Part model, mm, in its own coordinate system. A direction names the side the tool comes from. Give positions to 0.01 mm unless a question says otherwise; leave off trailing zeros. Write each loop counter-clockwise with the first axis right and the second up, starting at its lowest first coordinate (ties: lowest second). Pieces come first, ordered by that corner, then holes.
from build123d import *

# Parameters (mm, degrees)
F0_W     = 725
F0_H     = 620
F1_DEPTH = 2
F2_W     = 0.25
F2_H     = 110
F3_DEPTH = 25
F4_DEPTH = 25
F2_W_2   = 110
F2_H_2   = 0.2
F2_W_3   = 0.2
F2_H_3   = 399.6
F5_DEPTH = 25
F2_W_4   = 64.7
F6_DEPTH = 25
F2_W_5   = 45.1
F7_DEPTH = 25
F2_H_4   = 49.5626640439
F8_DEPTH = 25
F2_H_5   = 109.4
F2_W_6   = 9.8
F2_H_6   = 30.4373359561
F2_W_7   = 10
F2_H_7   = 29.8
F9_DEPTH = 25


# Not quite as in the source:
# - a feature names something its author has since deleted; it is built from what else it names


with BuildPart() as f1:
    # F0 (on Top) → F1 (new body)
    with BuildSketch(Plane.XY):
        with Locations((362.5, 310)):
            Rectangle(F0_W, F0_H)
    extrude(amount=F1_DEPTH)

    # F2 (on face) → F3 (join)
    with BuildSketch(Plane.XY.offset(2)):
        with Locations((614.875, 565)):
            Rectangle(F2_W, F2_H)
        with Locations((110.125, 565)):
            Rectangle(F2_W, F2_H)
        Polygon((110.2, 110), (110, 110), (110, 0), (110.25, 0), (110.25, 110), align=None)
        Polygon((615, 110), (614.8, 110), (614.75, 110), (614.75, 0), (615, 0), align=None)
    extrude(amount=-F3_DEPTH)

    # F2 (on face) → F4 (join)
    with BuildSketch(Plane.XY.offset(2)):
        Polygon((110, 510), (0, 510), (0, 509.8), (45.1, 509.8), (45.3, 509.8), (110, 509.8), align=None)
        Polygon((614.75, 510), (110.25, 510), (110.25, 509.8), (614.8, 509.8), (615, 509.8), (615, 510), align=None)
    extrude(amount=F4_DEPTH)

    # F2 (on face) → F5 (join)
    with BuildSketch(Plane.XY.offset(2)):
        with Locations((670, 509.9)):
            Rectangle(F2_W_2, F2_H_2)
        with Locations((614.9, 310)):
            Rectangle(F2_W_3, F2_H_3)
    extrude(amount=F5_DEPTH)

    # F2 (on face) → F6 (join)
    with BuildSketch(Plane.XY.offset(2)):
        with Locations((670, 110.1)):
            Rectangle(F2_W_2, F2_H_2)
        Polygon((614.8, 110.2), (110.2, 110.2), (110.2, 110), (110.25, 110), (614.75, 110), (614.8, 110), align=None)
        with Locations((614.9, 110.1)):
            Rectangle(F2_W_3, F2_H_2)
        with Locations((77.65, 110.1)):
            Rectangle(F2_W_4, F2_H_2)
        with Locations((110.1, 110.1)):
            Rectangle(F2_W_3, F2_H_2)
    extrude(amount=F6_DEPTH)

    # F2 (on face) → F7 (join)
    with BuildSketch(Plane.XY.offset(2)):
        with Locations((22.55, 110.1)):
            Rectangle(F2_W_5, F2_H_2)
    extrude(amount=F7_DEPTH)

    # F2 (on face) → F8 (join)
    with BuildSketch(Plane.XY.offset(2)):
        with Locations((45.2, 165.418667978)):
            Rectangle(F2_W_3, F2_H_4)
    extrude(amount=F8_DEPTH)

    # F2 (on face) → F9 (join)
    with BuildSketch(Plane.XY.offset(2)):
        Polygon((110.25, 510), (110, 510), (110, 509.8), (110.2, 509.8), (110.25, 509.8), align=None)
        with Locations((110.1, 310)):
            Rectangle(F2_W_3, F2_H_3)
        with Locations((45.2, 455.1)):
            Rectangle(F2_W_3, F2_H_5)
        with Locations((45.2, 400.3)):
            Rectangle(F2_W_3, F2_H_2)
        with Locations((40.2, 400.3)):
            Rectangle(F2_W_6, F2_H_2)
        with Locations((45.2, 125.418667978)):
            Rectangle(F2_W_3, F2_H_6)
        with Locations((45.2, 110.1)):
            Rectangle(F2_W_3, F2_H_2)
        with Locations((50.3, 400.3)):
            Rectangle(F2_W_7, F2_H_2)
        with Locations((45.2, 385.3)):
            Rectangle(F2_W_3, F2_H_7)
        with Locations((45.2, 165.418667978)):
            Rectangle(F2_W_3, F2_H_4)
        with Locations((45.2, 370.3)):
            Rectangle(F2_W_3, F2_H_2)
        with Locations((40.2, 370.3)):
            Rectangle(F2_W_6, F2_H_2)
        with Locations((40.2, 190.3)):
            Rectangle(F2_W_6, F2_H_2)
        with Locations((45.2, 190.3)):
            Rectangle(F2_W_3, F2_H_2)
        with Locations((50.3, 370.3)):
            Rectangle(F2_W_7, F2_H_2)
        with Locations((50.3, 190.3)):
            Rectangle(F2_W_7, F2_H_2)
        with Locations((45.2, 355.3)):
            Rectangle(F2_W_3, F2_H_7)
        with Locations((45.2, 205.3)):
            Rectangle(F2_W_3, F2_H_7)
        with Locations((45.2, 340.3)):
            Rectangle(F2_W_3, F2_H_2)
        with Locations((40.2, 340.3)):
            Rectangle(F2_W_6, F2_H_2)
        with Locations((40.2, 220.3)):
            Rectangle(F2_W_6, F2_H_2)
        with Locations((45.2, 220.3)):
            Rectangle(F2_W_3, F2_H_2)
        with Locations((50.3, 340.3)):
            Rectangle(F2_W_7, F2_H_2)
        with Locations((50.3, 220.3)):
            Rectangle(F2_W_7, F2_H_2)
        with Locations((45.2, 325.3)):
            Rectangle(F2_W_3, F2_H_7)
        with Locations((45.2, 235.3)):
            Rectangle(F2_W_3, F2_H_7)
        with Locations((45.2, 310.3)):
            Rectangle(F2_W_3, F2_H_2)
        with Locations((40.2, 310.3)):
            Rectangle(F2_W_6, F2_H_2)
        with Locations((40.2, 250.3)):
            Rectangle(F2_W_6, F2_H_2)
        with Locations((45.2, 250.3)):
            Rectangle(F2_W_3, F2_H_2)
        with Locations((50.3, 310.3)):
            Rectangle(F2_W_7, F2_H_2)
        with Locations((50.3, 250.3)):
            Rectangle(F2_W_7, F2_H_2)
        with Locations((45.2, 295.3)):
            Rectangle(F2_W_3, F2_H_7)
        with Locations((45.2, 265.3)):
            Rectangle(F2_W_3, F2_H_7)
        with Locations((45.2, 280.3)):
            Rectangle(F2_W_3, F2_H_2)
        with Locations((40.2, 280.3)):
            Rectangle(F2_W_6, F2_H_2)
        with Locations((50.3, 280.3)):
            Rectangle(F2_W_7, F2_H_2)
    extrude(amount=F9_DEPTH)


solid = f1.part
1) Saw through at D-D (y = 50). Write the cut outline in (x, z).
Check result:
outline: (0, 0) - (110, 0) - (110, -23) - (110.25, -23) - (110.25, 0) - (614.75, 0) - (614.75, -23) - (615, -23) - (615, 0) - (725, 0) - (725, 2) - (0, 2) - close
2) Flat gauge pins, fed straight in: P1, Ø5, axis at x = 49.5, z = 16.5, coming from the -Y side; P2, Ø7.5, axis at y = 211, z = 19.5, coming from the -X side; P3, Ø8, axis at y = 140.5, z = -0.5, coming from the -X side; P4, Ø3, axis at x = 353.5, z = 7, coming from the +Y side. Where does each tip first touch, or does it go through?
Check result:
P1: stops at y = 110
P2: stops at x = 45.1
P3: stops at x = 0
P4: stops at y = 510
3) Saw through at C-C (x = 458). Write the cut outline in (y, z).
Check result:
outline: (0, 0) - (620, 0) - (620, 2) - (510, 2) - (510, 27) - (509.8, 27) - (509.8, 2) - (110.2, 2) - (110.2, 27) - (110, 27) - (110, 2) - (0, 2) - close
4) Saw through at B-B (y = 379). Write the cut outline in (x, z), and give its area (4 significant figures).
Check result:
outline: (0, 0) - (725, 0) - (725, 2) - (615, 2) - (615, 27) - (614.8, 27) - (614.8, 2) - (110.2, 2) - (110.2, 27) - (110, 27) - (110, 2) - (45.3, 2) - (45.3, 27) - (45.1, 27) - (45.1, 2) - (0, 2) - close
area: 1,465 mm2
5) Drill centre lines: L1, parallel to X at y = 335.5, z = 7; L2, parallel to Y at x = 144, z = 15.5; L3, parallel to Z at x = 134.5, y = 504. Where is each one in solid material? Low to high.
Check result:
L1: x = 45.1 to 45.3, 110 to 110.2, 614.8 to 615
L2: y = 110 to 110.2, 509.8 to 510
L3: z = 0 to 2
6) 3-axis set-ups, long thin cutter, end or side, ignore diameter. For faces 5 (the flat face through (45.1, 386, 14)), 6 (the flat face through (78, 110.2, 14)), 7 (the flat face through (615, 54, -11)), 8 (the flat face through (671, 110.2, 14)): which of +Z, -Z, +X, -X, +Y, -Y reach the whole face in a straight line?
Check result:
face 5: +Z, -X
face 6: +Z
face 7: -Z, +X, +Y, -Y
face 8: +Z, +X
7) Mould opens along Y. For faces 1 (the flat face through (361, 620, 1)), 2 (the flat face through (359, 313, 2)), 3 (the flat face through (45.1, 205, 14)), 4 (the flat face through (725, 308.6, 0.4)) say: +Y half, -Y half, draft (parallel to the pull), parting line (faces both ways), or undercut.
Check result:
face 1: +Y half
face 2: undercut
face 3: undercut
face 4: draft
8) Saw through at A-A (z = -7.5). Write the cut outline in (x, y), and give its area (3 significant figures).
Check result:
outline: (110, 0) - (110.25, 0) - (110.25, 110) - (110, 110) - close; (110, 510) - (110.25, 510) - (110.25, 620) - (110, 620) - close; (614.75, 0) - (615, 0) - (615, 110) - (614.75, 110) - close; (614.75, 510) - (615, 510) - (615, 620) - (614.75, 620) - close
area: 110 mm2
